from build123d import *

# Parameters (mm, degrees)
SKETCH1_R           = 1.8
SKETCH1_R_2         = 1.6
SKETCH1_R_3         = 2.5
BOSS_EXTRUDE1_DEPTH = 6


with BuildPart() as part:
    # Sketch1 → Boss-Extrude1 (new body)
    with BuildSketch(Plane.XY):
        with BuildLine():
            Line((-157.361082537, 14.788780041), (-27.569235339, 144.58062724))
            ThreePointArc((-27.569235339, 144.58062724), (-21.080768362, 148.916082266), (-13.427099715, 150.438491616))
            Line((-13.427099715, 150.438491616), (78.999307156, 150.438491616))
            ThreePointArc((78.999307156, 150.438491616), (86.652975803, 148.916082266), (93.14144278, 144.58062724))
            Line((93.14144278, 144.58062724), (120.92318871, 116.798881309))
            ThreePointArc((120.92318871, 116.798881309), (125.258643737, 110.310414333), (126.781053087, 102.656745685))
            Line((126.781053087, 102.656745685), (126.781053087, 10.230338814))
            ThreePointArc((126.781053087, 10.230338814), (125.258643737, 2.576670167), (120.92318871, -3.91179681))
            Line((120.92318871, -3.91179681), (-8.868658488, -133.703644008))
            ThreePointArc((-8.868658488, -133.703644008), (-15.357125464, -138.039099034), (-23.010794112, -139.561508384))
            Line((-23.010794112, -139.561508384), (-104.123492484, -139.561508384))
            ThreePointArc((-104.123492484, -139.561508384), (-111.777161131, -138.039099034), (-118.265628108, -133.703644008))
            Line((-118.265628108, -133.703644008), (-157.361082537, -94.608189578))
            ThreePointArc((-157.361082537, -94.608189578), (-161.696537564, -88.119722602), (-163.218946913, -80.466053955))
            Line((-163.218946913, -80.466053955), (-163.218946913, 0.646644418))
            ThreePointArc((-163.218946913, 0.646644418), (-161.696537564, 8.300313065), (-157.361082537, 14.788780041))
        make_face()
        with Locations((-142.055996009, -95.771140482)):
            Circle(SKETCH1_R, mode=Mode.SUBTRACT)
        with Locations((-119.428579011, -118.39855748)):
            Circle(SKETCH1_R, mode=Mode.SUBTRACT)
        with Locations((87.753707876, 134.038563403)):
            Circle(SKETCH1_R, mode=Mode.SUBTRACT)
        with Locations((110.381124874, 111.411146405)):
            Circle(SKETCH1_R, mode=Mode.SUBTRACT)
        with Locations((23.240162175, 129.629094103)):
            Circle(SKETCH1_R_2, mode=Mode.SUBTRACT)
        with Locations((-59.491331224, 46.897600704)):
            Circle(SKETCH1_R_2, mode=Mode.SUBTRACT)
        with Locations((105.971655573, 46.897600704)):
            Circle(SKETCH1_R_2, mode=Mode.SUBTRACT)
        with Locations((23.240162175, -35.833892695)):
            Circle(SKETCH1_R_2, mode=Mode.SUBTRACT)
        with Locations((-153.35684456, -53.357593559)):
            Circle(SKETCH1_R_2, mode=Mode.SUBTRACT)
        with Locations((-75.57509863, -131.13933949)):
            Circle(SKETCH1_R_2, mode=Mode.SUBTRACT)
        with Locations((-105.639996778, -9.150559787)):
            Circle(SKETCH1_R_2, mode=Mode.SUBTRACT)
        with Locations((-32.807998316, -81.982558249)):
            Circle(SKETCH1_R_2, mode=Mode.SUBTRACT)
        with Locations((1.486680571, -47.687879362)):
            Circle(SKETCH1_R_2, mode=Mode.SUBTRACT)
        with Locations((-71.345317891, 25.144119101)):
            Circle(SKETCH1_R_2, mode=Mode.SUBTRACT)
        with Locations((-136.045588369, -70.66884975)):
            Circle(SKETCH1_R_2, mode=Mode.SUBTRACT)
        with Locations((-94.326288279, -112.38814984)):
            Circle(SKETCH1_R_2, mode=Mode.SUBTRACT)
        with Locations((-74.173745015, -92.235606576)):
            Circle(SKETCH1_R_2, mode=Mode.SUBTRACT)
        with Locations((-115.893045105, -50.516306486)):
            Circle(SKETCH1_R_2, mode=Mode.SUBTRACT)
        with Locations((-5.23083385, -98.246014216)):
            Circle(SKETCH1_R_2, mode=Mode.SUBTRACT)
        with Locations((17.396583148, -75.618597218)):
            Circle(SKETCH1_R_2, mode=Mode.SUBTRACT)
        with Locations((25.715035909, 141.296355992)):
            Circle(SKETCH1_R_2, mode=Mode.SUBTRACT)
        with Locations((117.638917463, 49.372474438)):
            Circle(SKETCH1_R_2, mode=Mode.SUBTRACT)
        with Locations((-88.218946913, 59.889285105)):
            Circle(SKETCH1_R_3, mode=Mode.SUBTRACT)
        with Locations((-88.218946913, 44.889285105)):
            Circle(SKETCH1_R_3, mode=Mode.SUBTRACT)
        with BuildLine():
            Line((-118.72147223, -10.211219959), (-97.508268795, -31.424423394))
            ThreePointArc((-97.508268795, -31.424423394), (-97.508268795, -45.566559018), (-111.650404418, -45.566559018))
            Line((-111.650404418, -45.566559018), (-132.863607854, -24.353355582))
            ThreePointArc((-132.863607854, -24.353355582), (-132.863607854, -10.211219959), (-118.72147223, -10.211219959))
        make_face(mode=Mode.SUBTRACT)
        with BuildLine():
            Line((-55.081861923, -73.850830265), (-33.868658488, -95.064033701))
            ThreePointArc((-33.868658488, -95.064033701), (-33.868658488, -109.206169325), (-48.010794112, -109.206169325))
            Line((-48.010794112, -109.206169325), (-69.223997547, -87.992965889))
            ThreePointArc((-69.223997547, -87.992965889), (-69.223997547, -73.850830265), (-55.081861923, -73.850830265))
        make_face(mode=Mode.SUBTRACT)
        Polygon((-6.998600803, -89.407179452), (3.608000915, -100.013781169), (19.164350101, -84.457431983), (8.557748383, -73.850830265), align=None, mode=Mode.SUBTRACT)
    extrude(amount=BOSS_EXTRUDE1_DEPTH)


solid = part.part
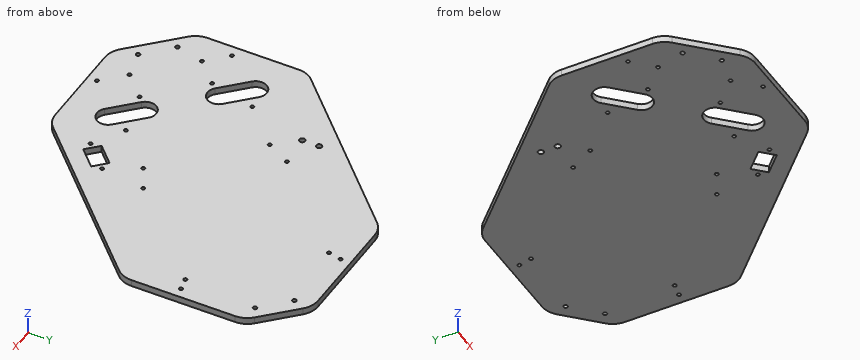
Check sheet for the modelled part. Datum: model origin and axes. Units: mm. Give positions to 0.01 mm unless a question says otherwise; leave off trailing zeros. Write each loop counter-clockwise with the first axis right and the second up, starting at its lowest first coordinate (ties: lowest second). Pieces come first, ordered by that corner, then holes. Notation, with made-up numbers: (0, 66) -> (56, 66) arc R5 ccw to (56, 74) -> close; hole circle Ø9 at (-20, 63). An arc over 180 degrees is marked (long way). Write item = value, one per line.
Item 1: Sectioned sample at C-C on y = 91. Record the boundary of the cut face in (x, z).
Output:
outline = (-81.15, 0) -> (126.78, 0) -> (126.78, 6) -> (-81.15, 6) -> close
Item 2: Sectioned sample at A-A on x = -125. Record the boundary of the cut face in (y, z), and give its area (3 significant figures).
Output:
outline = (-126.97, 0) -> (-32.22, 0) -> (-32.22, 6) -> (-126.97, 6) -> close; (-7.31, 0) -> (47.15, 0) -> (47.15, 6) -> (-7.31, 6) -> close
area = 895 mm^2
Item 3: Scan lines: probe 1 along Y at (x, z) = (-87.5, 3.6); probe 2 along Y at (x, z) = (-33.5, 0.3); probe 3 along X at (y, z) = (34.5, 2.6). Record each from-to range of solid material in increasing order. Write a range as from..to.
Output:
probe_1 = -139.56..42.49, 47.28..57.49, 62.28..84.65
probe_2 = -139.56..-108.82, -95.45..-83.43, -80.54..138.65
probe_3 = -137.65..126.78
Item 4: Sectioned sample at B-B on z = 4.55. Count the separate pieces of the cut face and the enclosed holes in it, and give its area (3 significant figures).
Output:
separate_pieces = 1
enclosed_holes = 27
area = 59,600 mm^2
Item 5: Sectioned sample at D-D on x = 33. Record the boundary of the cut face in (y, z).
Output:
outline = (-91.83, 0) -> (150.44, 0) -> (150.44, 6) -> (-91.83, 6) -> close
Item 6: Gauge pin test, flat ends, axial feed: pin 1 (3 mm diameter, centred on x = -153.36, y = -53.36, fed in from -Z); pin 2 (1 mm diameter, centred on x = -107, z = 4, fed in from -Y). Record the tip position at first contact, or that the pin passes through.
Output:
pin_1 = through
pin_2 = -139.42
